```python
from build123d import *

# Parameters (mm, degrees)
SKETCH1_R        = 10
EXTRUSION1_DEPTH = 5
HOLE1_D          = 2


with BuildPart() as part:
    # Sketch1 → Extrusion1 (new body)
    with BuildSketch(Plane(origin=(0, 0, 0), x_dir=(-1, 0, 0), z_dir=(0, 1, 0))):
        with Locations(Location((0, 0, 0), (0, 0, 90))):
            Circle(SKETCH1_R)
        with BuildLine():
            ThreePointArc((1.2, 1.6), (-2, 0), (1.2, -1.6))
            Line((1.2, -1.6), (3.2, -1.6))
            Line((3.2, -1.6), (3.2, 1.6))
            Line((3.2, 1.6), (1.2, 1.6))
        make_face(mode=Mode.SUBTRACT)
    extrude(amount=EXTRUSION1_DEPTH)

    # Hole1 (through all)
    with Locations(Plane(origin=(0, 5, 0), x_dir=(1, 0, 0), z_dir=(0, 1, 0))):
        with Locations((0, -5.5), (0, 5.5)):
            Hole(HOLE1_D / 2)


solid = part.part
```
The model under review builds one solid part; all positions refer to its coordinate system, in mm. A direction names the side the tool comes from. Coordinates: 2 decimals unless noted, no trailing zeros. Loops run counter-clockwise (first coordinate to the right, second up) from the corner with the lowest first, then second, coordinate; pieces in that order, holes last. Notation, with made-up numbers: (29.25, -25) -> (83.25, -25) arc R33 ccw to (83.25, 14) -> close; hole circle Ø8 at (-5, 8). An arc over 180 degrees is marked (long way). Answer as CSV lines item,"result".
Item 1: Draft analysis for pull direction Z (two halves, no side actions). For faces 3 (the flat face through (2.4, 5, -0.1)), 4 (the cylindrical face through (2, 2, 0)), 5 (the cylindrical face through (-9.76, 2.46, -2.17)), state which applies: +Z half, -Z half, draft (parallel to the pull), parting line (faces both ways), or undercut.
Results below:
face 3,"draft"
face 4,"undercut"
face 5,"parting line"
Item 2: Take a section at A-A, the plane z = -6.25. State the section outline as (x, y) points, and give its area (3 significant figures).
Results below:
outline,"(-7.81, 0) -> (-0.66, 0) -> (-0.66, 5) -> (-7.81, 5) -> close; (0.66, 0) -> (7.81, 0) -> (7.81, 5) -> (0.66, 5) -> close"
area,"71.4 mm2"
Item 3: Take a section at B-B, the plane y = 1.75. State the section outline as (x, z) points, and give its area (3 significant figures).
Results below:
outline,"circle Ø20 at (0, 0); hole (-3.2, -1.6) -> (-1.2, -1.6) arc R2 ccw (long way) to (-1.2, 1.6) -> (-3.2, 1.6) -> close; hole circle Ø2 at (0, -5.5); hole circle Ø2 at (0, 5.5)"
area,"291 mm2"
Item 4: Take a section at D-D, the plane z = 0. State the section outline as (x, y) points, and give its area (3 significant figures).
Results below:
outline,"(-10, 0) -> (-3.2, 0) -> (-3.2, 5) -> (-10, 5) -> close; (2, 0) -> (10, 0) -> (10, 5) -> (2, 5) -> close"
area,"74.0 mm2"
Item 5: Machinability: for faces 1 (the flat face through (-2, 2, -1.6)), 2 (the flat face through (2.4, 0, -0.1)), which of the approach directions +Z, -Z, +X, -X, +Y, -Y give a long, thin tool a straight path to every point of the face, cutting with its end or side? Answer none if there is none.
Results below:
face 1,"+Y, -Y"
face 2,"+Z, -Z, +X, -X, -Y"
Item 6: Insertion check: pin 1 (1.6 mm diameter, centred on x = -2, y = 2.5, fed in from +Z); pin 2 (3 mm diameter, centred on y = 3.5, z = 5, fed in from -X); pin 3 (1.6 mm diameter, centred on x = -2, y = 3.5, fed in from -Z). Each pin has a flat end and moves straight along its axis. Give the tip position at first contact, or say it passes through.
Results below:
pin 1,"stops at z = 9.93"
pin 2,"stops at x = -9.37"
pin 3,"stops at z = -9.93"
Item 7: For L1, parallel to X at y = 3.25, z = -5.5; L2, parallel to X at y = 3.9, z = -0.25; L3, parallel to Z at x = 3, y = 4.8, list the stretches that pass through material, from the lowest coordinate up.
Results below:
L1,"x = -8.35 to -1, 1 to 8.35"
L2,"x = -10 to -3.2, 1.98 to 10"
L3,"z = -9.54 to 9.54"
Item 8: Take a section at C-C, the plane x = -0.75. State the section outline as (y, z) points.
Results below:
outline,"(0, -9.97) -> (5, -9.97) -> (5, -6.16) -> (0, -6.16) -> close; (0, -4.84) -> (5, -4.84) -> (5, -1.85) -> (0, -1.85) -> close; (0, 1.85) -> (5, 1.85) -> (5, 4.84) -> (0, 4.84) -> close; (0, 6.16) -> (5, 6.16) -> (5, 9.97) -> (0, 9.97) -> close"
